from build123d import *

# Parameters (mm, degrees)
F0_W     = 300
F0_H     = 300
F1_DEPTH = 300
F2_R     = 20
F3_R     = 25
F4_DEPTH = 30
F5_R     = 25
F6_DEPTH = 3


with BuildPart() as f1:
    # F0 (on Top) → F1 (new body)
    with BuildSketch(Plane.XY):
        with Locations((-64.879608, 0.722477)):
            Rectangle(F0_W, F0_H)
    extrude(amount=F1_DEPTH)

    # F2
    f2_edges = [f1.edges().sort_by_distance(p)[0] for p in [
        (-214.879608, 150.722477, 150),
        (-64.879608, 150.722477, 300),
        (-214.879608, 0.722477, 300),
        (-64.879608, 150.722477, 0),
        (-214.879608, 0.722477, 0),
        (-64.879608, -149.277523, 0),
        (85.120392, 0.722477, 0),
        (85.120392, 150.722477, 150),
        (-214.879608, -149.277523, 150),
        (85.120392, -149.277523, 150),
        (-64.879608, -149.277523, 300),
        (85.120392, 0.722477, 300),
    ]]
    fillet(f2_edges, radius=F2_R)

    # F3 (on face) → F4 (cut)
    with BuildSketch(Plane(origin=(0, 0, 0), x_dir=(1, 0, 0), z_dir=(0, 0, -1))):
        with Locations((-64.879608, -0.722477)):
            Circle(F3_R)
    extrude(amount=-F4_DEPTH, mode=Mode.SUBTRACT)

    # F5 (on face) → F6 (cut)
    with BuildSketch(Plane(origin=(-214.879608, 0, 0), x_dir=(0, -1, 0), z_dir=(-1, 0, 0))):
        with Locations((64.277523, 215)):
            Circle(F5_R)
        with Locations((-0.722477, 150)):
            Circle(F5_R)
        with Locations((64.277523, 85)):
            Circle(F5_R)
        with Locations((-65.722477, 85)):
            Circle(F5_R)
        with Locations((-65.722477, 215)):
            Circle(F5_R)
    extrude(amount=-F6_DEPTH, mode=Mode.SUBTRACT)


solid = f1.part
Geometry: final body of the model. Coordinates: model frame, mm. A direction names the side the tool comes from. Give positions to 0.01 mm unless a question says otherwise; leave off trailing zeros. Write each loop counter-clockwise with the first axis right and the second up, starting at its lowest first coordinate (ties: lowest second). Pieces come first, ordered by that corner, then holes.
(1) Cut plane A-A, the plane y = -9. Return loops of the section in (x, z).
(2) Access query for faces 1 (the cylindrical face through (-41.034, -6.787, 14.79)), 2 (the cylindrical face through (-213.401, -61.023, 239.787)), 3 (the cylindrical face through (-209.18, -143.26, 151.82)). Directions: +Z, -Z, +X, -X, +Y, -Y. A direction counts if a zero-diameter tool reaches every point of the face in a straight line with its end or side. Return the directions, or none.
(3) Ray query, line 1 (X direction, y = 84.5, z = 95.5); line 2 (Z direction, x = -198, y = 88.5); line 3 (X direction, y = -134.5, z = 275.5). Return the intervals inside material, ascending.
(4) First-contact query: P1, Ø25, axis at x = -65, y = 0, coming from the -Z side; P2, Ø15, axis at y = 60, z = 225.5, coming from the -X side. Flat tips, straight axial feed; report the tip coordinate or a pass-through.
(5) Mould query, pull axis Z, two halves, no side actions, for faces 4 (the flat face through (-211.88, 66, 85)), 5 (the flat face through (-38, 3, 0)), 6 (the cylindrical face through (-63.06, 145.019, 293.986)). Classes: released by +Z, released by -Z, zero draft, split by the parting line, or undercut.
Values follow:
1. outline: (-214.88, 20) arc R20 ccw to (-194.88, 0) - (-87.91, 0) - (-87.91, 30) - (-41.85, 30) - (-41.85, 0) - (65.12, 0) arc R20 ccw to (85.12, 20) - (85.12, 280) arc R20 ccw to (65.12, 300) - (-194.88, 300) arc R20 ccw to (-214.88, 280) - (-214.88, 173.03) - (-211.88, 173.03) - (-211.88, 126.97) - (-214.88, 126.97) - close
2. face 1: -Z
2. face 2: -X
2. face 3: +Z, -Z, -X, -Y
3. line 1: x = -211.88 to 85.12
3. line 2: z = 0.24 to 299.76
3. line 3: x = -214.19 to 84.43
4. P1: stops at z = 30
4. P2: stops at x = -211.88
5. face 4: undercut
5. face 5: released by -Z
5. face 6: released by +Z
